CAD build for the part. Positions are in the model's coordinates, mm. Face numbers are marked on the shaded views. Give positions to 0.01 mm unless a question says otherwise; leave off trailing zeros. Loops run counter-clockwise (first coordinate to the right, second up) from the corner with the lowest first, then second, coordinate; pieces in that order, holes last.
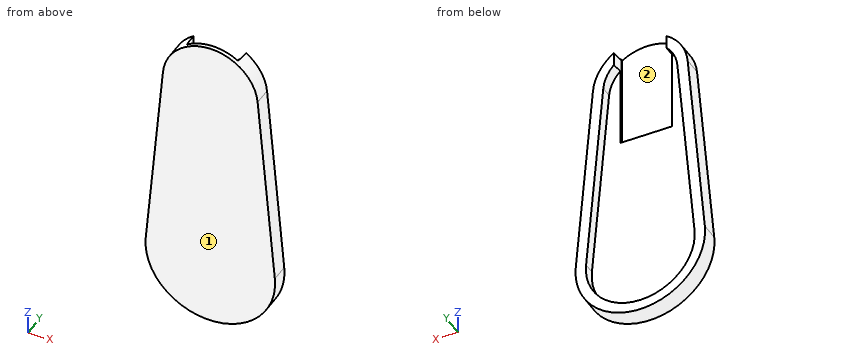
Autodesk Inventor part; units mm, degrees
ref_plane "YZ Plane" through (0, 0, 0) normal (1, 0, 0) x (0, 1, 0)
ref_plane "XZ Plane" through (0, 0, 0) normal (0, 1, 0) x (-1, 0, 0)
ref_plane "XY Plane" through (0, 0, 0) normal (0, 0, 1) x (1, 0, 0)
sketch "Sketch1" plane through (0, 0, 0) normal (0, 1, 0) x (-1, 0, 0)
  arc A0 (5.4799, 0.7804) -> (-5.4769, 0.7804) centre (0.0015, 0.2935) ccw
  arc A1 (-7.4691, -21.6354) -> (7.472, -21.6354) centre (0.0015, -22.2993) ccw
  line L0 (-5.4769, 0.7804) -> (-7.4691, -21.6354)
  line L1 (5.4799, 0.7804) -> (7.472, -21.6354)
  line L2 (6.2767, -21.7416) -> (4.2846, 0.6742)
  arc A2 (4.2846, 0.6742) -> (-4.2816, 0.6742) centre (0.0015, 0.2935) ccw
  line L3 (-4.2816, 0.6742) -> (-6.2738, -21.7416)
  arc A3 (-6.2738, -21.7416) -> (6.2767, -21.7416) centre (0.0015, -22.2993) ccw
  dimension "d18" = 11
  dimension "d19" = 15
  dimension "d22" = 1.2
extrude "Extrusion7" add sketch "Sketch1" along normal blind 2.1
extrude "Extrusion8" add sketch "Sketch1" along normal blind 0.8 contours A3 L3 A2 L2
sketch "Sketch5" plane through (0, 0, 0) normal (0, 0, 1) x (1, 0, 0)
  line L0 (-3.019, 0.8) -> (2.981, 0.8)
  line L1 (5.4769, 0) -> (-5.4799, 0)
  line L2 (-3.019, 0.8) -> (-3.019, 4.3274)
  line L3 (-3.019, 4.3274) -> (3.2255, 4.3274)
  line L4 (3.2255, 4.3274) -> (2.981, 0.8)
  point P0 (0, 0)
  point P1 (-0.0015, 0)
  dimension "d27" = 6
  dimension "d28" = 0.8
extrude "Extrusion9" cut sketch "Sketch5" along normal blind 14.7
sketch "Sketch6" plane through (0, 0.8, 0) normal (0, 1, 0) x (1, 0, 0)
  line L0 (-2.99, -5.9206) -> (2.938, -5.9206)
  line L1 (2.938, -5.9206) -> (2.938, 6.0287)
  line L2 (2.938, 6.0287) -> (-2.99, 6.0287)
  line L3 (-2.99, 6.0287) -> (-2.99, -5.9206)
  point P0 (0, 0)
extrude "Extrusion10" cut sketch "Sketch6" against normal blind 0.3
properties part number "Tapa1_3DPrint"
1. Saw through at D-D, the plane z = -2.5. List the corners of the cut face in (x, y).
Responses:
outline: (-5.77, 0) - (5.77, 0) - (5.77, 2.1) - (4.56, 2.1) - (4.56, 0.8) - (2.94, 0.8) - (2.94, 0.5) - (-2.99, 0.5) - (-2.99, 0.8) - (-4.57, 0.8) - (-4.57, 2.1) - (-5.77, 2.1) - close
2. Saw through at C-C, the plane y = 1.65. List the corners of the cut face in (x, z).
Responses:
outline: (-7.47, -21.64) arc R7.5 ccw (long way) to (7.47, -21.64) - (5.48, 0.78) arc R5.5 ccw to (3.04, 4.88) - (3.04, 3.33) arc R4.3 cw to (4.28, 0.67) - (6.27, -21.74) arc R6.3 cw (long way) to (-6.28, -21.74) - (-4.28, 0.67) arc R4.3 cw to (-3.02, 3.36) - (-3.02, 4.89) arc R5.5 ccw to (-5.48, 0.78) - close
3. Probe line 1 along Y through (x, z) = (-4.5, -16); line 2 along X through (y, z) = (1.85, -23); line 3 along X through (y, z) = (1.2, -6). List the from-to ranges inside material, lowest first.
Responses:
line 1: y = 0 to 0.8
line 2: x = -7.47 to -6.26, 6.26 to 7.47
line 3: x = -6.08 to -4.88, 4.87 to 6.08
4. Drop flat-ended pins along their axis: pin 1 (2 mm diameter, centred on x = 1, z = -3, fed in from +Y); pin 2 (1 mm diameter, centred on x = -5, y = 0.5, fed in from +Z). Give the stop position or say it passes through.
Responses:
pin 1: stops at y = 0.5
pin 2: stops at z = 3.46
5. Saw through at B-B, the plane x = -0.5. List the corners of the cut face in (y, z), and give its area (3 significant figures).
Responses:
outline: (0, -29.78) - (2.1, -29.78) - (2.1, -28.58) - (0.8, -28.58) - (0.8, -6.03) - (0.5, -6.03) - (0.5, 5.77) - (0, 5.77) - close
area: 26.5 mm2
6. Pull direction X, two halves, no side cores. Call the marked faces 1 and 2: released by +X, released by -X, zero draft, split by the parting line, or undercut.
Responses:
face 1: zero draft
face 2: undercut
7. Saw through at A-A, the plane z = -23.5. List the corners of the cut face in (x, y), and give its area (3 significant figures).
Responses:
outline: (-7.4, 0) - (7.4, 0) - (7.4, 2.1) - (6.18, 2.1) - (6.18, 0.8) - (-6.19, 0.8) - (-6.19, 2.1) - (-7.4, 2.1) - close
area: 15.0 mm2
